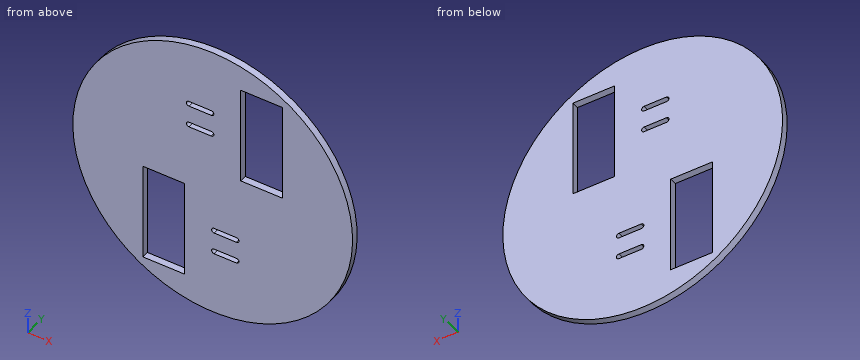
from build123d import *

# Parameters (mm, degrees)
SKETCH_1_R               = 100
EXTRUDE_1_DEPTH          = 5
SKETCH_3_W               = 30
SKETCH_3_H               = 70
CUT_EXTRUDE_1_DEPTH      = 142.509716981
CUT_EXTRUDE_2_DEPTH      = 142.509716981
PATTERN_CIRCULAR_1_COUNT = 2


with BuildPart() as part:
    # 草图1 → 凸台-拉伸1 (new body)
    with BuildSketch(Plane(origin=(0, 0, 0), x_dir=(1, 0, 0), z_dir=(0, 1, 0))):
        with Locations(Location((0, 0, 0), (0, 0, 270))):
            Circle(SKETCH_1_R)
    extrude(amount=EXTRUDE_1_DEPTH)

    # 草图3 → 切除-拉伸1 (cut, through all)
    with BuildSketch(Plane(origin=(0, 0, 0), x_dir=(1, 0, 0), z_dir=(0, 1, 0))):
        with Locations((35, -45)):
            Rectangle(SKETCH_3_W, SKETCH_3_H)
    cut_extrude_1 = extrude(amount=CUT_EXTRUDE_1_DEPTH, mode=Mode.SUBTRACT)

    # 草图2 → 切除-拉伸2 (cut, through all)
    with BuildSketch(Plane(origin=(0, 0, 0), x_dir=(1, 0, 0), z_dir=(0, 1, 0))):
        with BuildLine():
            Line((-17, -35.2), (-1, -35.2))
            ThreePointArc((-1, -35.2), (0.8, -37), (-1, -38.8))
            Line((-1, -38.8), (-17, -38.8))
            ThreePointArc((-17, -38.8), (-18.8, -37), (-17, -35.2))
        make_face()
        with BuildLine():
            Line((-17, -54.8), (-1, -54.8))
            ThreePointArc((-1, -54.8), (0.8, -53), (-1, -51.2))
            Line((-1, -51.2), (-17, -51.2))
            ThreePointArc((-17, -51.2), (-18.8, -53), (-17, -54.8))
        make_face()
    cut_extrude_2 = extrude(amount=CUT_EXTRUDE_2_DEPTH, mode=Mode.SUBTRACT)

    # 阵列(圆周)1: 切除-拉伸1, 切除-拉伸2 ×2 about axis
    pattern_circular_1_axis = Axis((0, 0, 0), (0, 1, 0))
    add([cut_extrude_1.rotate(pattern_circular_1_axis, i * 360 / PATTERN_CIRCULAR_1_COUNT) for i in range(1, PATTERN_CIRCULAR_1_COUNT)], mode=Mode.SUBTRACT)
    add([cut_extrude_2.rotate(pattern_circular_1_axis, i * 360 / PATTERN_CIRCULAR_1_COUNT) for i in range(1, PATTERN_CIRCULAR_1_COUNT)], mode=Mode.SUBTRACT)


solid = part.part
Geometry check sheet. Reference: the model listing, model coordinates, mm. Round coordinates to 2 decimals unless told otherwise and drop trailing zeros. Order: outer loops, then holes, each group sorted by start corner. A loop starts at its lowest first (then second) coordinate and runs counter-clockwise, first axis right, second up. Notation, with made-up numbers: M -37,14.5 L 20,14.5 A16 ccw 20,36.5 Z; hole C -39,80 d5. An arc over 180 degrees is marked long. Answer in a Markdown table with one row per item.
(1) Go/stop test with flat-tipped pins: P1, Ø2.5, axis at x = 28.5, y = 1.5, coming from the -Z side; P2, Ø1.5, axis at x = 28, y = 3, coming from the +Z side; P3, Ø1.5, axis at y = 3.5, z = -50, coming from the -X side. Record where each tip stops, or that it passes through.
Responses:
| item | result |
|---|---|
| P1 | stops at z = -96.22 |
| P2 | stops at z = 96.22 |
| P3 | stops at x = -87.03 |
(2) Sectioned sample at A-A, the plane z = -73. Record the cut outline in (x, y), and give its area (3 significant figures).
Responses:
| item | result |
|---|---|
| outline | M -68.34,0 L -50,0 L -50,5 L -68.34,5 Z; M -20,0 L 68.34,0 L 68.34,5 L -20,5 Z |
| area | 533 mm² |
(3) Sectioned sample at B-B, the plane x = 39.5. Record the cut outline in (y, z), and give its area (3 significant figures).
Responses:
| item | result |
|---|---|
| outline | M 0,-91.87 L 5,-91.87 L 5,10 L 0,10 Z; M 0,80 L 5,80 L 5,91.87 L 0,91.87 Z |
| area | 569 mm² |
(4) Scan lines: probe 1 along Z at (x, y) = (2, 0.7); probe 2 along Z at (x, y) = (-13, 2.35); probe 3 along Z at (x, y) = (23.5, 2.35). Record each from-to range of solid material in increasing order. Write a range as from..to.
Responses:
| item | result |
|---|---|
| probe 1 | z = -99.98..-54.8, -51.2..-38.8, -35.2..99.98 |
| probe 2 | z = -99.15..35.2, 38.8..51.2, 54.8..99.15 |
| probe 3 | z = -97.2..10, 80..97.2 |
(5) Sectioned sample at C-C, the plane y = 2.2. Record the cut outline in (x, z), and give its area (3 significant figures).
Responses:
| item | result |
|---|---|
| outline | C 0,0 d200; hole M -50,-80 L -20,-80 L -20,-10 L -50,-10 Z; hole M -17,35.2 L -1,35.2 A1.8 ccw -1,38.8 L -17,38.8 A1.8 ccw Z; hole M -17,51.2 L -1,51.2 A1.8 ccw -1,54.8 L -17,54.8 A1.8 ccw Z; hole M 1,-54.8 L 17,-54.8 A1.8 ccw 17,-51.2 L 1,-51.2 A1.8 ccw Z; hole M 1,-38.8 L 17,-38.8 A1.8 ccw 17,-35.2 L 1,-35.2 A1.8 ccw Z; hole M 20,10 L 50,10 L 50,80 L 20,80 Z |
| area | 26,900 mm² |
(6) Sectioned sample at D-D, the plane x = 74.5. Record the cut outline in (y, z).
Responses:
| item | result |
|---|---|
| outline | M 0,-66.71 L 5,-66.71 L 5,66.71 L 0,66.71 Z |
